For this review, use the dimensioned drawing (mm, ordinates from the lowest corner) and the shaded views. A direction names the side the tool comes from. Round coordinates to 2 decimals unless told otherwise and drop trailing zeros. Write each loop counter-clockwise with the first axis right and the second up, starting at its lowest first coordinate (ties: lowest second). Pieces come first, ordered by that corner, then holes. Notation, with made-up numbers: M 56.5,48 L 87.5,48 A22 cw 87.5,77 Z; hole C -15,56.5 d1. An arc over 180 degrees is marked long. Answer in a Markdown table with one row per item.
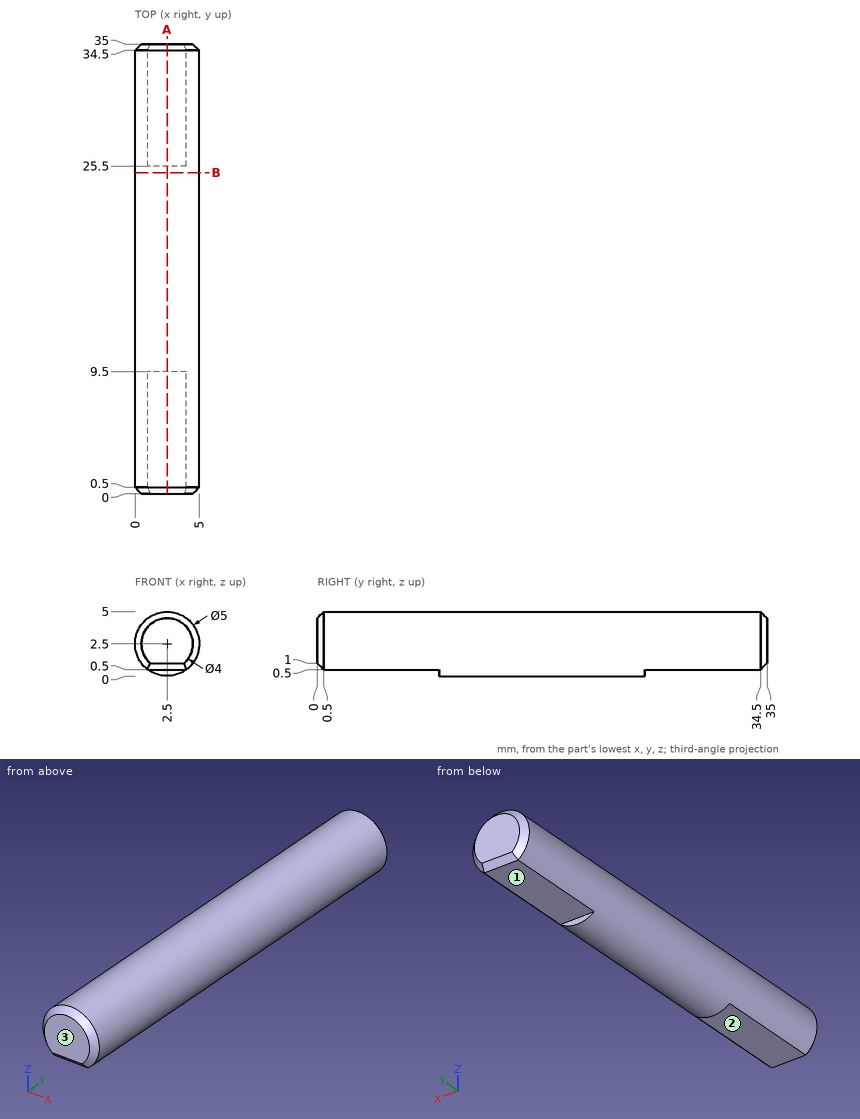
Q1. For probe 1 along Z at (x, y) = (4.5, 4.5); probe 2 along Z at (x, y) = (2.4, 13); probe 3 along X at (y, z) = (23, 3.75) (1 decimal), list the stretches that pass through material, from the lowest coordinate up.
Found:
| item | result |
|---|---|
| probe 1 | 1 to 4 |
| probe 2 | 0 to 5 |
| probe 3 | 0.3 to 4.7 |
Q2. Take a section at B-B (y = 25). State the section outline as (x, z) points, then the cut area to 3 significant figures.
Found:
| item | result |
|---|---|
| outline | C 2.5,2.5 d5 |
| area | 19.6 mm² |
Q3. Take a section at A-A (x = 2.5). State the section outline as (y, z) points.
Found:
| item | result |
|---|---|
| outline | M 0,1 L 0.5,0.5 L 9.5,0.5 L 9.5,0 L 25.5,0 L 25.5,0.5 L 34.5,0.5 L 35,1 L 35,4.5 L 34.5,5 L 0.5,5 L 0,4.5 Z |
Q4. Insertion check: P1, Ø2, axis at y = 13, z = 4.5, coming from the -X side; P2, Ø1.5, axis at x = 2, y = 5.5, coming from the -Z side. Each pin has a flat end and moves straight along its axis. Give the tip position at first contact, or say it passes through.
Found:
| item | result |
|---|---|
| P1 | x = 0.21 |
| P2 | z = 0.5 |
Q5. Machinability: for the marked faces 1, 2 and 3, which of the approach directions +Z, -Z, +X, -X, +Y, -Y give a long, thin tool a straight path to every point of the face, cutting with its end or side? Answer none if there is none.
Found:
| item | result |
|---|---|
| face 1 | -Z, +X, -X, +Y |
| face 2 | -Z, +X, -X, -Y |
| face 3 | +Z, -Z, +X, -X, -Y |
